Geometry check sheet. Reference: the model listing, model coordinates, mm. A direction names the side the tool comes from. Round coordinates to 2 decimals unless told otherwise and drop trailing zeros. Order: outer loops, then holes, each group sorted by start corner. A loop starts at its lowest first (then second) coordinate and runs counter-clockwise, first axis right, second up. Notation, with made-up numbers: (74, 73.25) - (116, 73.25) arc R26 ccw to (116, 100.25) - close; hole circle Ø10 at (-20, -35.5). An arc over 180 degrees is marked (long way). Write each question's results on one line, items separated by ' | '.
```python
from build123d import *

# Parameters (mm, degrees)
SKETCH1_W          = 230
SKETCH1_H          = 230
SKETCH1_W_2        = 170
SKETCH1_H_2        = 170
BORDER_DEPTH       = 6
SKETCH2_R          = 3
CUT_EXTRUDE1_DEPTH = 326.324453431
FILLET1_R          = 1


with BuildPart() as part:
    # Sketch1 → border (new body)
    with BuildSketch(Plane(origin=(0, 0, 0), x_dir=(1, 0, 0), z_dir=(0, 1, 0))):
        with Locations((115, 115)):
            Rectangle(SKETCH1_W, SKETCH1_H)
        with Locations((115, 115)):
            Rectangle(SKETCH1_W_2, SKETCH1_H_2, mode=Mode.SUBTRACT)
    extrude(amount=BORDER_DEPTH)

    # Sketch2 → Cut-Extrude1 (cut, through all)
    with BuildSketch(Plane(origin=(0, 6, 0), x_dir=(1, 0, 0), z_dir=(0, 1, 0))):
        with Locations(Location((10, 220, 0), (0, 0, 270))):
            Circle(SKETCH2_R)
        with Locations(Location((220, 220, 0), (0, 0, 270))):
            Circle(SKETCH2_R)
        with Locations(Location((220, 10, 0), (0, 0, 270))):
            Circle(SKETCH2_R)
        with Locations(Location((10, 10, 0), (0, 0, 270))):
            Circle(SKETCH2_R)
    extrude(amount=-CUT_EXTRUDE1_DEPTH, mode=Mode.SUBTRACT)

    # Fillet1
    fillet1_edges = [part.edges().sort_by_distance(p)[0] for p in [
        (30, 3, -200),
        (30, 3, -30),
        (200, 3, -30),
        (200, 3, -200),
        (0, 3, -230),
        (230, 3, -230),
        (230, 3, 0),
        (0, 3, 0),
    ]]
    fillet(fillet1_edges, radius=FILLET1_R)


solid = part.part
```
(1) Section check C-C (z = -35.5). Record the cut outline in (x, y).
Answers follow:
outline: (0, 0) - (30, 0) - (30, 6) - (0, 6) - close; (200, 0) - (230, 0) - (230, 6) - (200, 6) - close
(2) Material ranges on line 1 (X direction, y = 4.2, z = -220); line 2 (X direction, y = 3.4, z = -84.5); line 3 (Z direction, x = 220, y = 3.4), recorded low to high.
Answers follow:
line 1: 0 to 7, 13 to 217, 223 to 230 | line 2: 0 to 30, 200 to 230 | line 3: -230 to -223, -217 to -13, -7 to 0
(3) Access from +Z, -Z, +X, -X, +Y, -Y to the whole of each face (thin tool, end or side, straight path). Record for faces 1 (the face through (114, 3, -200)), 2 (the face through (230, 3, -113)).
Answers follow:
face 1: +Y, -Y | face 2: +Z, -Z, +X, +Y, -Y
(4) Depth check by flat-ended pin: pin 1 Ø5.5 at (x, z) = (10, -220) entering from -Y. Enter the tip coordinate at first touch or a pass-through.
Answers follow:
pin 1: through
(5) Section check D-D (y = 1.4). Record the cut outline in (x, z).
Answers follow:
outline: (0, -229) arc R1 ccw to (1, -230) - (229, -230) arc R1 ccw to (230, -229) - (230, -1) arc R1 ccw to (229, 0) - (1, 0) arc R1 ccw to (0, -1) - close; hole circle Ø6 at (10, -220); hole circle Ø6 at (10, -10); hole (30, -199) arc R1 ccw to (31, -200) - (199, -200) arc R1 ccw to (200, -199) - (200, -31) arc R1 ccw to (199, -30) - (31, -30) arc R1 ccw to (30, -31) - close; hole circle Ø6 at (220, -220); hole circle Ø6 at (220, -10)
(6) Draft check along Z on faces 3 (the face through (113, 0, -14)), 4 (the face through (113, 3, 0)), 5 (the face through (223, 3, -10)). Enter one of: released by +Z, released by -Z, zero draft, split by the parting line, or undercut.
Answers follow:
face 3: zero draft | face 4: released by +Z | face 5: undercut
(7) Section check B-B (x = 153). Record the cut outline in (y, z), then the cut area to 3 significant figures.
Answers follow:
outline: (0, -230) - (6, -230) - (6, -200) - (0, -200) - close; (0, -30) - (6, -30) - (6, 0) - (0, 0) - close | area: 360 mm²
(8) Section check A-A (x = 10). Record the cut outline in (y, z).
Answers follow:
outline: (0, -230) - (6, -230) - (6, -223) - (0, -223) - close; (0, -217) - (6, -217) - (6, -13) - (0, -13) - close; (0, -7) - (6, -7) - (6, 0) - (0, 0) - close
